from build123d import *

# Parameters (mm, degrees)
SKETCH1_R           = 1.5
SKETCH1_R_2         = 1
BOSS_EXTRUDE1_DEPTH = 1.6
SKETCH3_W           = 30.784918317
SKETCH3_H           = 1.24969352
CUT_EXTRUDE2_DEPTH  = 10


with BuildPart() as part:
    # Sketch1 → Boss-Extrude1 (new body)
    with BuildSketch(Plane.XY):
        with BuildLine():
            Line((-9.5, -11.5), (9.5, -11.5))
            ThreePointArc((9.5, -11.5), (10.914213562, -10.914213562), (11.5, -9.5))
            Line((11.5, -9.5), (11.5, 9.5))
            ThreePointArc((11.5, 9.5), (10.914213562, 10.914213562), (9.5, 11.5))
            Line((9.5, 11.5), (-9.5, 11.5))
            ThreePointArc((-9.5, 11.5), (-10.914213562, 10.914213562), (-11.5, 9.5))
            Line((-11.5, 9.5), (-11.5, -9.5))
            ThreePointArc((-11.5, -9.5), (-10.914213562, -10.914213562), (-9.5, -11.5))
        make_face()
        Circle(SKETCH1_R, mode=Mode.SUBTRACT)
        with Locations((9, 9)):
            Circle(SKETCH1_R_2, mode=Mode.SUBTRACT)
        with Locations(Location((-9, 9, 0), (0, 0, 180))):
            Circle(SKETCH1_R_2, mode=Mode.SUBTRACT)
        with Locations((-9, -9)):
            Circle(SKETCH1_R_2, mode=Mode.SUBTRACT)
        with Locations(Location((9, -9, 0), (0, 0, 180))):
            Circle(SKETCH1_R_2, mode=Mode.SUBTRACT)
    extrude(amount=BOSS_EXTRUDE1_DEPTH)

    # Sketch3 → Cut-Extrude2 (cut)
    with BuildSketch(Plane(origin=(0, 0, 0), x_dir=(-1, 0, 0), z_dir=(0, 0, -1))):
        with Locations((-2.857529043, 11.62484676)):
            Rectangle(SKETCH3_W, SKETCH3_H)
    extrude(amount=-CUT_EXTRUDE2_DEPTH, mode=Mode.SUBTRACT)


solid = part.part
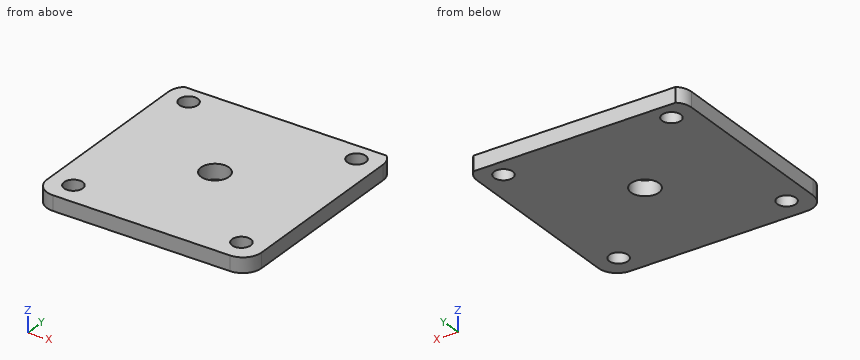
Verification items for the finished model (mm, model axes). Coordinates: 2 decimals unless noted, no trailing zeros. Order: outer loops, then holes, each group sorted by start corner. A loop starts at its lowest first (then second) coordinate and runs counter-clockwise, first axis right, second up. Notation, with made-up numbers: (-34.75, -7) -> (-2.75, -7) arc R20 cw to (-2.75, 8) -> close; hole circle Ø6 at (50, -11.75). An arc over 180 degrees is marked (long way). Use CSV: the item, a comma, the result in double quotes. Start each with the question number.
Q1. Depth check by flat-ended pin: P1, Ø1.2, axis at x = -9, y = -9, coming from the -Z side. Enter the tip coordinate at first touch or a pass-through.
Q2. Section check B-B, the plane x = 9. Record the cut outline in (y, z), and give its area (3 significant figures).
Q3. Section check C-C, the plane z = 0.5. Record the cut outline in (x, y).
Q4. Section check A-A, the plane y = 9. Record the cut outline in (x, z).
Q5. Thickness scan on line 1 along Y through (x, z) = (-9, 0.35); line 2 along X through (y, z) = (-9.5, 1.05); line 3 along Y through (x, z) = (-1.25, 0.8). Record the ranges inside material, lowest first.
Returned:
1,P1,"passes through"
2,outline,"(-11.5, 0) -> (-10, 0) -> (-10, 1.6) -> (-11.5, 1.6) -> close; (-8, 0) -> (8, 0) -> (8, 1.6) -> (-8, 1.6) -> close; (10, 0) -> (11, 0) -> (11, 1.6) -> (10, 1.6) -> close"
2,area,"29.6 mm^2"
3,outline,"(-11.5, -9.5) arc R2 ccw to (-9.5, -11.5) -> (9.5, -11.5) arc R2 ccw to (11.5, -9.5) -> (11.5, 9.5) arc R2 ccw to (10.82, 11) -> (-10.82, 11) arc R2 ccw to (-11.5, 9.5) -> close; hole circle Ø2 at (-9, -9); hole circle Ø2 at (-9, 9); hole circle Ø3 at (0, 0); hole circle Ø2 at (9, -9); hole circle Ø2 at (9, 9)"
4,outline,"(-11.5, 0) -> (-10, 0) -> (-10, 1.6) -> (-11.5, 1.6) -> close; (-8, 0) -> (8, 0) -> (8, 1.6) -> (-8, 1.6) -> close; (10, 0) -> (11.5, 0) -> (11.5, 1.6) -> (10, 1.6) -> close"
5,line 1,"y = -11.5 to -10, -8 to 8, 10 to 11"
5,line 2,"x = -11.5 to -9.87, -8.13 to 8.13, 9.87 to 11.5"
5,line 3,"y = -11.5 to -0.83, 0.83 to 11"
